from build123d import *

# Parameters (mm, degrees)
ESQUISSE1_W               = 650
ESQUISSE1_H               = 900
T_LE_DE_BASE_PLI_E1_DEPTH = 2
ESQUISSE6_W               = 500
ESQUISSE6_H               = 10
ENL_V_MAT_EXTRU_1_DEPTH   = 10
ESQUISSE7_R               = 25
BOSS_EXTRU_1_DEPTH        = 20
ESQUISSE8_R               = 35
BOSS_EXTRU_2_DEPTH        = 20
CONG_1_R                  = 5
ESQUISSE9_R               = 2.5
ENL_V_MAT_EXTRU_2_DEPTH   = 20


# Sheet-metal steps are written as plain solids
with BuildPart() as part:
    # Esquisse1 → Tôle de base pliée1 (new body)
    with BuildSketch(Plane.XY):
        Rectangle(ESQUISSE1_W, ESQUISSE1_H)
    extrude(amount=-T_LE_DE_BASE_PLI_E1_DEPTH)

    # Esquisse6 → Enlèv. mat.-Extru.1 (cut)
    with BuildSketch(Plane.XY):
        with Locations((0, 345)):
            Rectangle(ESQUISSE6_W, ESQUISSE6_H)
        with Locations((0, 305)):
            Rectangle(ESQUISSE6_W, ESQUISSE6_H)
        with Locations((0, 265)):
            Rectangle(ESQUISSE6_W, ESQUISSE6_H)
        with Locations((0, 225)):
            Rectangle(ESQUISSE6_W, ESQUISSE6_H)
        with Locations((0, 185)):
            Rectangle(ESQUISSE6_W, ESQUISSE6_H)
        with Locations((0, 145)):
            Rectangle(ESQUISSE6_W, ESQUISSE6_H)
        with Locations((0, 105)):
            Rectangle(ESQUISSE6_W, ESQUISSE6_H)
        with Locations((0, 65)):
            Rectangle(ESQUISSE6_W, ESQUISSE6_H)
    extrude(amount=-ENL_V_MAT_EXTRU_1_DEPTH, mode=Mode.SUBTRACT)

    # Esquisse7 → Boss.-Extru.1 (add)
    with BuildSketch(Plane.XY):
        with Locations((250, 0)):
            Circle(ESQUISSE7_R)
    extrude(amount=BOSS_EXTRU_1_DEPTH)

    # Esquisse8 → Boss.-Extru.2 (add)
    with BuildSketch(Plane.XY.offset(20)):
        with Locations((250, 0)):
            Circle(ESQUISSE8_R)
    extrude(amount=BOSS_EXTRU_2_DEPTH)

    # Congé1
    cong_1_edges = [part.edges().sort_by_distance(p)[0] for p in [
        (225, 0, 0),
        (225, 0, 20),
        (215, 0, 40),
    ]]
    fillet(cong_1_edges, radius=CONG_1_R)

    # Esquisse9 → Enlèv. mat.-Extru.2 (cut)
    with BuildSketch(Plane.XY):
        with Locations((-312.5, 243.775317496)):
            Circle(ESQUISSE9_R)
        with Locations((-312.5, 227.775317496)):
            Circle(ESQUISSE9_R)
        with Locations((-312.5, 211.775317496)):
            Circle(ESQUISSE9_R)
        with Locations((-312.5, -36.224682504)):
            Circle(ESQUISSE9_R)
        with Locations((-312.5, -52.224682504)):
            Circle(ESQUISSE9_R)
        with Locations((-312.5, -68.224682504)):
            Circle(ESQUISSE9_R)
        with Locations((-312.5, -316.224682504)):
            Circle(ESQUISSE9_R)
        with Locations((-312.5, -332.224682504)):
            Circle(ESQUISSE9_R)
        with Locations((-312.5, -348.224682504)):
            Circle(ESQUISSE9_R)
    extrude(amount=-ENL_V_MAT_EXTRU_2_DEPTH, mode=Mode.SUBTRACT)


solid = part.part
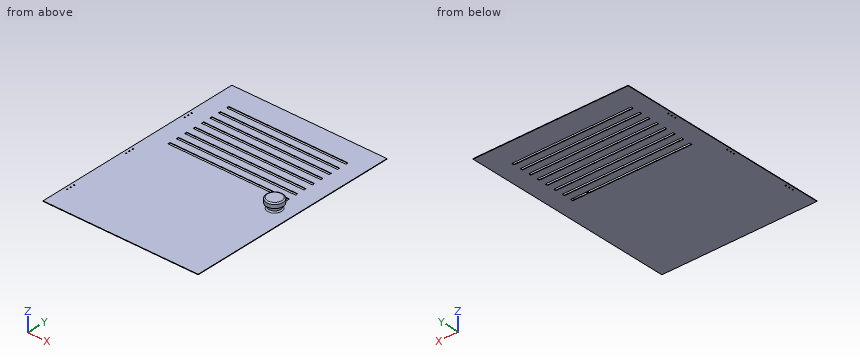
The listing builds one solid part. Answer for the finished solid, in the listing's coordinates (mm). Round coordinates to 2 decimals unless told otherwise and drop trailing zeros. Loops run counter-clockwise (first coordinate to the right, second up) from the corner with the lowest first, then second, coordinate; pieces in that order, holes last. Notation, with made-up numbers: M 11.5,-26 L 31.5,-26 A35 ccw 31.5,6 Z; hole C 64,63 d5. An arc over 180 degrees is marked long. Write each question's results on one line, items separated by ' | '. Start each with the question number.
1) Each of these flat-tipped pins is pushed along its axis until it touches: pin 1 (3 mm diameter, centred on x = -312.5, y = 211.78, fed in from +Z); pin 2 (8 mm diameter, centred on x = -251, y = -255, fed in from +Z). Where does it stop, or does it pass through?
2) Find section B-B on x = -198. Count the separate pieces of the cut face and the enclosed holes in it, plus the area to 3 significant figures.
3) Find section C-C on y = -100. Write down the section's boundary in (x, z).
4) Straight lines are drawn through the part: probe 1 along Z at (x, y) = (224, -309.5); probe 2 along Y at (x, z) = (244.5, 23); probe 3 along X at (y, z) = (11.5, 10). For each, find the intervals that lie inside material, in ascending order.
5) Find section A-A on y = 0. Write down the section's boundary in (x, z).
Final values:
1) pin 1: through | pin 2: z = 0
2) separate pieces: 9 | enclosed holes: 0 | area: 1,640 mm²
3) outline: M -325,-2 L 325,-2 L 325,0 L -325,0 Z
4) probe 1: -2 to 0 | probe 2: -34.57 to 34.57 | probe 3: 227.8 to 272.2
5) outline: M -325,-2 L 325,-2 L 325,0 L 280,0 A5 cw 275,5 L 275,15 A5 cw 280,20 L 285,20 L 285,35 A5 ccw 280,40 L 220,40 A5 ccw 215,35 L 215,20 L 220,20 A5 cw 225,15 L 225,5 A5 cw 220,0 L -325,0 Z
